The model under review builds one solid part; all positions refer to its coordinate system, in mm. A direction names the side the tool comes from. Round coordinates to 2 decimals unless told otherwise and drop trailing zeros. Loops run counter-clockwise (first coordinate to the right, second up) from the corner with the lowest first, then second, coordinate; pieces in that order, holes last. Notation, with made-up numbers: (-37, 68.5) -> (-18, 68.5) arc R17 cw to (-18, 101.5) -> close; hole circle Ø8 at (22, 9.25). An arc over 180 degrees is marked (long way). Use a Markdown table: item, result. Add a question column.
1) Wall thickness on probe 1 along Z at (x, y) = (0, -21) (3 decimals); probe 2 along Y at (x, z) = (0, 5.5); probe 3 along X at (y, z) = (-8.5, 9): over which ranges is each line inside the solid? List them lowest first.
2) Consider section B-B on y = -16. Give the boundary of the cut face in (x, z), plus the area to 3 significant figures.
3) Mouldability with a two-part tool opening along X and no side actions: class faces 4 (the cylindrical face through (-4.76, 11.893, 3.451)), 5 (the flat face through (10.5, -9, 10)), 6 (the flat face through (0, -23, 36.195)) as released by +X, released by -X, zero draft, split by the parting line, or undercut.
4) For faces 1 (the flat face through (0, 19.05, 3)), 2 (the flat face through (-8.5, -12, 11)), 3 (the flat face through (-9.486, -14.626, 10.161)), list the 3-axis set-ups (+Z, -Z, +X, -X, +Y, -Y) from which the entire face can be reached by the end or side of a thin tool; tool diameter is ignored.
5) Consider section C-C on z = 30.5. Give the boundary of the cut face in (x, y).
6) Insertion check: pin 1 (2 mm diameter, centred on x = 0, y = 9.805, fed in from -Z); pin 2 (4 mm diameter, centred on x = 5.5, z = 21.5, fed in from +Y); pin 3 (4 mm diameter, centred on x = -3.5, z = 27, fed in from +Y); pin 4 (4.5 mm diameter, centred on x = -5.58, y = -13.47, fed in from +Z). Each pin has a flat end and moves straight along its axis. Give the tip position at first contact, or say it passes through.
7) Consider section A-A on x = 5.58. Give the boundary of the cut face in (y, z) (3 decimals), plus the area to 3 significant figures.
8) Consider section D-D on x = 0. Give the boundary of the cut face in (y, z) (3 decimals), plus the area to 3 significant figures.
from build123d import *

# Parameters (mm, degrees)
SKETCH1_W           = 21
SKETCH1_H           = 38.1
SKETCH1_R           = 1.778
BOSS_EXTRUDE1_DEPTH = 7
SKETCH3_W           = 21
SKETCH3_H           = 7
BOSS_EXTRUDE2_DEPTH = 36.195
SKETCH4_R           = 2
CUT_EXTRUDE1_DEPTH  = 10.5
BOSS_EXTRUDE3_DEPTH = 2
BOSS_EXTRUDE4_START = -19
BOSS_EXTRUDE4_DEPTH = 2


with BuildPart() as part:
    # Sketch1 → Boss-Extrude1 (new body)
    with BuildSketch(Plane.XY):
        Rectangle(SKETCH1_W, SKETCH1_H)
        with Locations((-5.58, 13.47)):
            Circle(SKETCH1_R, mode=Mode.SUBTRACT)
        with Locations((5.58, 13.47)):
            Circle(SKETCH1_R, mode=Mode.SUBTRACT)
        with Locations((0, 9.805)):
            Circle(SKETCH1_R, mode=Mode.SUBTRACT)
        with Locations((5.58, -13.47)):
            Circle(SKETCH1_R, mode=Mode.SUBTRACT)
        with Locations((0, -9.805)):
            Circle(SKETCH1_R, mode=Mode.SUBTRACT)
        with Locations((-5.58, -13.47)):
            Circle(SKETCH1_R, mode=Mode.SUBTRACT)
    extrude(amount=BOSS_EXTRUDE1_DEPTH)

    # Sketch3 → Boss-Extrude2 (add)
    with BuildSketch(Plane(origin=(0, 0, 0), x_dir=(-1, 0, 0), z_dir=(0, 0, -1))):
        with Locations((0, -22.55)):
            Rectangle(SKETCH3_W, SKETCH3_H)
    extrude(amount=-BOSS_EXTRUDE2_DEPTH)

    # Sketch4 → Cut-Extrude1 (cut)
    with BuildSketch(Plane.XZ.offset(26.05)):
        with Locations((0, 13.195)):
            Circle(SKETCH4_R)
        with Locations((0, 29.195)):
            Circle(SKETCH4_R)
    extrude(amount=-CUT_EXTRUDE1_DEPTH, mode=Mode.SUBTRACT)

    # Sketch5 → Boss-Extrude3 (add)
    with BuildSketch(Plane(origin=(10.5, 0, 0), x_dir=(0, 0, -1), z_dir=(1, 0, 0))):
        Polygon((-18.0975, -26.05), (0, 0), (0, 7.197126675), (-23.0975, -26.05), align=None)
    extrude(amount=-BOSS_EXTRUDE3_DEPTH)

    # Sketch5<2> → Boss-Extrude4 (add)
    with BuildSketch(Plane(origin=(10.5, 0, 0), x_dir=(0, 0, -1), z_dir=(1, 0, 0)).offset(BOSS_EXTRUDE4_START)):
        Polygon((-18.0975, -26.05), (0, 0), (0, 7.197126675), (-23.0975, -26.05), align=None)
    extrude(amount=-BOSS_EXTRUDE4_DEPTH)


solid = part.part
Result set:
| question | item | result |
|---|---|---|
| 1 | probe 1 | 0 to 11.195, 15.195 to 27.195, 31.195 to 36.195 |
| 1 | probe 2 | -26.05 to -11.58, -8.03 to 8.03, 11.58 to 19.05 |
| 1 | probe 3 | -10.5 to -8.5, 8.5 to 10.5 |
| 2 | outline | (-10.5, 0) -> (10.5, 0) -> (10.5, 7) -> (-10.5, 7) -> close; (-10.5, 11.12) -> (-8.5, 11.12) -> (-8.5, 16.12) -> (-10.5, 16.12) -> close; (8.5, 11.12) -> (10.5, 11.12) -> (10.5, 16.12) -> (8.5, 16.12) -> close |
| 2 | area | 167 mm2 |
| 3 | face 4 | undercut |
| 3 | face 5 | released by +X |
| 3 | face 6 | zero draft |
| 4 | face 1 | +Z, -Z, +X, -X, +Y |
| 4 | face 2 | +Z, +Y |
| 4 | face 3 | +X, -X |
| 5 | outline | (-10.5, -26.05) -> (-1.52, -26.05) -> (-1.52, -19.05) -> (-10.5, -19.05) -> close; (1.52, -26.05) -> (10.5, -26.05) -> (10.5, -19.05) -> (1.52, -19.05) -> close |
| 6 | pin 1 | through |
| 6 | pin 2 | y = -19.05 |
| 6 | pin 3 | y = -19.05 |
| 6 | pin 4 | z = 7 |
| 7 | outline | (-26.05, 0) -> (-15.248, 0) -> (-15.248, 7) -> (-19.05, 7) -> (-19.05, 36.195) -> (-26.05, 36.195) -> close; (-11.692, 0) -> (11.692, 0) -> (11.692, 7) -> (-11.692, 7) -> close; (15.248, 0) -> (19.05, 0) -> (19.05, 7) -> (15.248, 7) -> close |
| 7 | area | 470 mm2 |
| 8 | outline | (-26.05, 0) -> (-11.583, 0) -> (-11.583, 7) -> (-19.05, 7) -> (-19.05, 11.195) -> (-26.05, 11.195) -> close; (-26.05, 15.195) -> (-19.05, 15.195) -> (-19.05, 27.195) -> (-26.05, 27.195) -> close; (-26.05, 31.195) -> (-19.05, 31.195) -> (-19.05, 36.195) -> (-26.05, 36.195) -> close; (-8.027, 0) -> (8.027, 0) -> (8.027, 7) -> (-8.027, 7) -> close; (11.583, 0) -> (19.05, 0) -> (19.05, 7) -> (11.583, 7) -> close |
| 8 | area | 414 mm2 |
